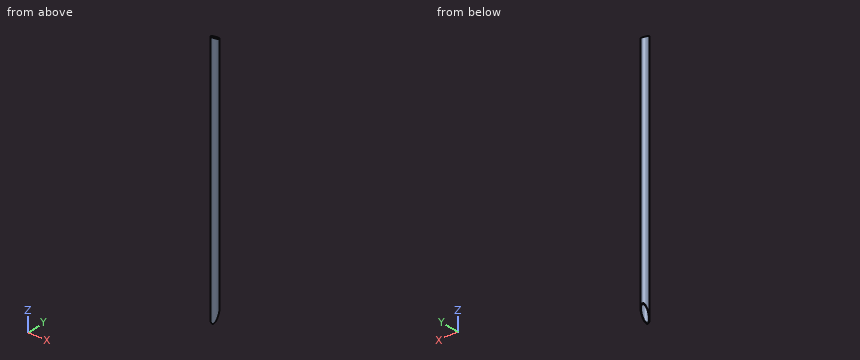
Autodesk Inventor part; units mm, degrees
ref_plane "Начальная плоскость" through (0, 0, 83.8147) normal (0, 0, 1) x (1, 0, 0)
ref_plane "Конечная плоскость" through (0, 0, 661.5922) normal (0, 0, 1) x (1, 0, 0)
ref_plane "РабПлоскость4" through (-8, 240.1857, 549.4966) normal (0, 0.4116224, 0.9113545) x (1, 0, 0)
ref_plane "Начальная плоскость" through (0, 0, 83.8147) normal (0, 0, 1) x (1, 0, 0)
ref_plane "Конечная плоскость" through (0, 0, 661.5922) normal (0, 0, 1) x (1, 0, 0)
sketch "Эскиз" plane through (0, 0, 0) normal (0, 0, 1) x (1, 0, 0)
  circle A0 centre (0, 0) radius 7
  circle A1 centre (0, 0) radius 8
  dimension "d0" = 16
  dimension "d1" = 1
extrude "Тело" add sketch "Эскиз" along normal up to surface (577.7775 mm away) from surface at 83.8147
sketch "Sketch3" plane through (0, 0, 0) normal (0, 0, 1) x (1, 0, 0)
  line L0 (0, 0) -> (10, 0)
ref_plane "Work Plane3" through (0, 0, 0) normal (0, -1, 0) x (1, 0, 0)
sketch "Sketch4" plane through (0, 0, 0) normal (0, -1, 0) x (1, 0, 0)
  line L0 (-2, 83.8147) -> (12, 83.8147)
  line L1 (-2, 661.5922) -> (12, 661.5922)
  dimension "d7" = 577.7775
ref_plane "РабПлоскость4" through (-8, 240.1857, 549.4966) normal (0, 0.4116224, 0.9113545) x (1, 0, 0)
split "Разделение1" plane through (-8, 240.1857, 549.4966) removes the side toward (0, 0.4116224, 0.9113545)
ref_plane "РабПлоскость5" through (-8, 209.5672, 565.5203) normal (0, 0.9113545, -0.4116224) x (1, 0, 0)
split "Разделение2" plane through (-8, 209.5672, 565.5203) removes the side toward (0, 0.9113545, -0.4116224)
equation "\"d0\" = G_H"
equation "\"d1\" = G_T"
equation "\"d2\" = G_L"
equation "\"G_H\" = 16"
equation "\"G_T\" = 1"
equation "\"G_L\" = d7"
equation "\"G_OFFSET_START\" = -83.81468"
equation "\"G_OFFSET_END\" = -2.19454"
equation "\"d4\" = -G_OFFSET_START"
equation "\"d5\" = G_OFFSET_END + B_L"
equation "\"B_L\" = 663.78672"
properties part number "Труба 16x1-577,78 ГОСТ 10704-91" material "Сталь, мягкая"
Work out the finished part from the listing and answer in its coordinate system (mm). Round coordinates to 2 decimals unless told otherwise and drop trailing zeros. Write each loop counter-clockwise with the first axis right and the second up, starting at its lowest first coordinate (ties: lowest second). Pieces come first, ordered by that corner, then holes. Notation, with made-up numbers: (39.25, -17) - (80.25, -17) arc R16 ccw to (80.25, 4) - close; hole circle Ø1 at (-28.75, 75). An arc over 180 degrees is marked (long way). Answer in a Markdown table with one row per item. Add a question column.
1. A cutting plane is placed at C-C, the plane z = 214.5. Determine the outline of the cut face in (x, y), and give its area (3 significant figures).
2. Find the intervals of material crossed by line 1 along X through (y, z) = (0, 411.5); line 2 along Y through (x, z) = (1.25, 341.5), in increasing order. Write a range as from..to.
3. A cutting plane is placed at B-B, the plane y = 0. Determine the outline of the cut face in (x, z), and give its area (3 significant figures).
4. A cutting plane is placed at A-A, the plane x = -4. Determine the outline of the cut face in (y, z), and give its area (3 significant figures).
5. Given pin 1 (1.5 mm diameter, centred on x = -0.5, z = 531.5, fed in from -Y); pin 2 (2 mm diameter, centred on y = 2.5, z = 159.5, fed in from +X); pin 3 (1 mm diameter, centred on y = -3, z = 595.5, fed in from -X); pin 4 (3 mm diameter, centred on x = 4, z = 600, fed in from -Y), each flat-ended and moving along its own axis, determine where each tip first touches the part or whether it passes through.
Worked out:
| question | item | result |
|---|---|---|
| 1 | outline | circle Ø16 at (0, 0); hole circle Ø14 at (0, 0) |
| 1 | area | 47.1 mm^2 |
| 2 | line 1 | -8..-7, 7..8 |
| 2 | line 2 | -7.9..-6.89, 6.89..7.9 |
| 3 | outline | (-8, 101.53) - (-7, 101.53) - (-7, 657.98) - (-8, 657.98) - close; (7, 101.53) - (8, 101.53) - (8, 657.98) - (7, 657.98) - close |
| 3 | area | 1,110 mm^2 |
| 4 | outline | (-6.93, 86.19) - (-5.74, 88.81) - (-5.74, 660.57) - (-6.93, 661.11) - close; (5.74, 114.25) - (6.93, 116.87) - (6.93, 654.85) - (5.74, 655.38) - close |
| 4 | area | 1,320 mm^2 |
| 5 | pin 1 | y = -8 |
| 5 | pin 2 | x = 7.86 |
| 5 | pin 3 | x = -7.6 |
| 5 | pin 4 | y = -7.6 |
